Work out the finished part from the listing and answer in its coordinate system (mm). A direction names the side the tool comes from. Coordinates: 2 decimals unless noted, no trailing zeros. Loops run counter-clockwise (first coordinate to the right, second up) from the corner with the lowest first, then second, coordinate; pieces in that order, holes last.
```python
from build123d import *

# Parameters (mm, degrees)
BOSS_EXTRUDE1_DEPTH = 6.35
SKETCH2_R           = 1.5875
SKETCH2_W           = 9.525
SKETCH2_H           = 12.0015
CUT_EXTRUDE1_DEPTH  = 6.35


with BuildPart() as part:
    # Sketch1 → Boss-Extrude1 (new body)
    with BuildSketch(Plane(origin=(0, 0, 0), x_dir=(0, 0, -1), z_dir=(1, 0, 0))):
        Polygon((-50.8, -28.575), (-50.8, -41.275), (-19.05, -41.275), (-19.05, -34.925), (19.05, -34.925), (19.05, -41.275), (50.8, -41.275), (50.8, -28.575), (44.45, -28.575), (44.45, 22.225), (50.8, 22.225), (50.8, 41.275), (19.05, 41.275), (19.05, 34.925), (-19.05, 34.925), (-19.05, 41.275), (-50.8, 41.275), (-50.8, 22.225), (-44.45, 22.225), (-44.45, -28.575), align=None)
    extrude(amount=BOSS_EXTRUDE1_DEPTH)

    # Sketch2 → Cut-Extrude1 (cut)
    with BuildSketch(Plane(origin=(6.35, 95.4107123, 69.821382876), x_dir=(0, 0, -1), z_dir=(1, 0, 0))):
        with Locations((90.458882876, -118.4294623)):
            Circle(SKETCH2_R)
        with Locations((90.458882876, -91.4419623)):
            Circle(SKETCH2_R)
        with Locations((90.458882876, -104.9357123)):
            Rectangle(SKETCH2_W, SKETCH2_H)
    extrude(amount=-CUT_EXTRUDE1_DEPTH, mode=Mode.SUBTRACT)


solid = part.part
```
1. For faces 5 (the flat face through (3, 22.225, 48)), 6 (the flat face through (3, -15.526, -21)), 7 (the flat face through (3, -38, -19.05)), 8 (the flat face through (3, 38, 19.05)), 9 (the flat face through (3, -28.575, -48)), determine the directions among +Z, -Z, +X, -X, +Y, -Y from which every point of the face is accessible in a straight line to the end or side of a thin tool.
2. Each of these flat-tipped pins is pushed along its axis until it touches: P1, Ø1, axis at x = 1.5, y = -27.5, coming from the +Z side; P2, Ø1.9, axis at x = 3, y = 7.5, coming from the -Z side; P3, Ø4, axis at y = 3.97, z = -20.64, coming from the +X side. Where does it stop, or does it pass through?
3. Determine the mould class of faces 1 (the flat face through (3, -3, 44.45)), 2 (the flat face through (3, -10, -15.875)), 3 (the flat face through (3, -38, 19.05)), 4 (the flat face through (3, -41.275, 35)) for opening direction Y: released by +Y, released by -Y, zero draft, split by the parting line, or undercut.
4. A cutting plane is placed at D-D, the plane y = 18. Give the vertices of the cut face in (x, z).
5. A cutting plane is placed at B-B, the plane x = 2. Count the separate pieces of the cut face and the enclosed holes in it, then the cut area to 3 significant figures.
6. A cutting plane is placed at A-A, the plane y = -13. Give the vertices of the cut face in (x, z) (3 decimals).
7. Straight lines are drawn through the part: probe 1 along Z at (x, y) = (0.5, -9.5) (3 decimals); probe 2 along Y at (x, z) = (4.25, -20) (3 decimals); probe 3 along Z at (x, y) = (5.25, 1.5). For each, find the intervals that lie inside material, in ascending order.
8. A cutting plane is placed at C-C, the plane z = -5.5. Give the vertices of the cut face in (x, y) (3 decimals).
Answers below:
1. face 5: +Z, +X, -X
1. face 6: +X, -X
1. face 7: +X, -X, -Y
1. face 8: +X, -X, +Y
1. face 9: -Z, +X, -X
2. P1: stops at z = 44.45
2. P2: stops at z = -44.45
2. P3: stops at x = 6.35
3. face 1: undercut
3. face 2: undercut
3. face 3: zero draft
3. face 4: released by -Y
4. outline: (0, -44.45) - (6.35, -44.45) - (6.35, 44.45) - (0, 44.45) - close
5. separate pieces: 1
5. enclosed holes: 3
5. area: 7,130 mm2
6. outline: (0, -44.45) - (6.35, -44.45) - (6.35, -25.4) - (0, -25.4) - close; (0, -15.875) - (6.35, -15.875) - (6.35, 44.45) - (0, 44.45) - close
7. probe 1: z = -44.45 to -25.4, -15.875 to 44.45
7. probe 2: y = -41.275 to -24.473, -21.565 to -15.526, -3.524 to 2.515, 5.423 to 41.275
7. probe 3: z = -44.45 to 44.45
8. outline: (0, -34.925) - (6.35, -34.925) - (6.35, 34.925) - (0, 34.925) - close
